Design review of the part shown in the three views and the two pictorial views. Dimensions are in mm from the part's minimum x, y and z. Round coordinates to 2 decimals unless told otherwise and drop trailing zeros. Loops run counter-clockwise (first coordinate to the right, second up) from the corner with the lowest first, then second, coordinate; pieces in that order, holes last. Notation, with made-up numbers: M 51,88.5 L 86,88.5 A23 cw 86,122.5 Z; hole C 31,77.25 d2. An arc over 180 degrees is marked long. Return JSON: item names as keys, results as strings. Group by question number.
Q1. To check wall thickness, follow line 1 along X through (y, z) = (8.25, 10); line 2 along Z through (x, y) = (8.25, 3.5); line 3 along X through (y, z) = (10.75, 21.75). State the ranges of each line that lie inside material, in increasing order.
Q2. Consider section C-C (x = 7.5). State the section outline as (y, z) points, and give its area (3 significant figures).
Q3. Consider section D-D (y = 18.25). State the section outline as (x, z) points.
Q4. Consider section A-A (z = 10). State the section outline as (x, y) points, and give its area (3 significant figures).
Q5. Consider section B-B (y = 10). State the section outline as (x, z) points.
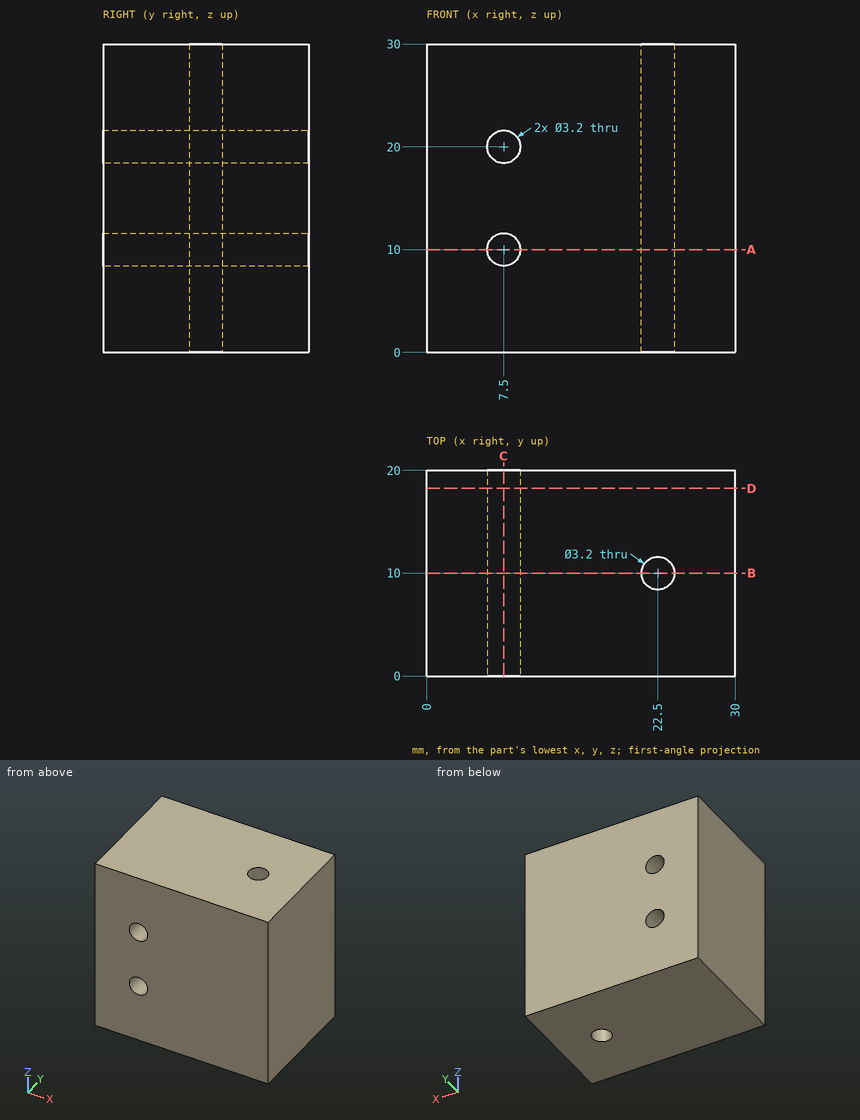
Values:
{
 "1": {"line 1": "x = 0 to 5.9, 9.1 to 30", "line 2": "z = 0 to 8.59, 11.41 to 18.59, 21.41 to 30", "line 3": "x = 0 to 21.09, 23.91 to 30"},
 "2": {"outline": "M 0,0 L 20,0 L 20,8.4 L 0,8.4 Z; M 0,11.6 L 20,11.6 L 20,18.4 L 0,18.4 Z; M 0,21.6 L 20,21.6 L 20,30 L 0,30 Z", "area": "472 mm2"},
 "3": {"outline": "M 0,0 L 30,0 L 30,30 L 0,30 Z; hole C 7.5,10 d3.2; hole C 7.5,20 d3.2"},
 "4": {"outline": "M 0,0 L 5.9,0 L 5.9,20 L 0,20 Z; M 9.1,0 L 30,0 L 30,20 L 9.1,20 Z; hole C 22.5,10 d3.2", "area": "528 mm2"},
 "5": {"outline": "M 0,0 L 20.9,0 L 20.9,30 L 0,30 Z; M 24.1,0 L 30,0 L 30,30 L 24.1,30 Z; hole C 7.5,10 d3.2; hole C 7.5,20 d3.2"}
}
